```python
from build123d import *

# Parameters (mm, degrees)
F1_DEPTH = 4
F2_R     = 5
F3_R     = 3.99999
F4_DEPTH = 3


# Not quite as in the source:
# - a fillet or chamfer is up to 0.001 mm smaller than in the source, because OpenCascade refuses the exact size
# - a feature names something its author has since deleted; it is built from what else it names


with BuildPart() as f1:
    # F0 (on Front) → F1 (new body)
    with BuildSketch(Plane.XZ):
        with BuildLine():
            Line((-4.5, -6.79), (-4.5, -2.79))
            Line((-4.5, -2.79), (-8, -2.79))
            ThreePointArc((-8, -2.79), (-10.5, -5.29), (-13, -2.79))
            Line((-13, -2.79), (-14.5, -2.79))
            Line((-14.5, -2.79), (-14.5, -6.79))
            Line((-14.5, -6.79), (-4.5, -6.79))
        make_face()
        with BuildLine():
            ThreePointArc((-13, -2.79), (-10.5, -5.29), (-8, -2.79))
            Line((-8, -2.79), (-13, -2.79))
        make_face()
        with BuildLine():
            Line((-3.5307081443, -2.79), (-4.5, -2.79))
            Line((-4.5, -2.79), (-4.5, -6.79))
            Line((-4.5, -6.79), (-3.5307081443, -6.79))
            ThreePointArc((-3.5307081443, -6.79), (-1.9615045246, -5.53), (0, -5.08))
            Line((0, -5.08), (0, -4.5))
            ThreePointArc((0, -4.5), (-1.9615045246, -4.05), (-3.5307081443, -2.79))
        make_face()
        with BuildLine():
            ThreePointArc((4.5, 0), (3.1819805153, 3.1819805153), (0, 4.5))
            ThreePointArc((0, 4.5), (-3.1819805153, 3.1819805153), (-4.5, 0))
            ThreePointArc((-4.5, 0), (-4.2507756145, -1.4767893131), (-3.5307081443, -2.79))
            Line((-3.5307081443, -2.79), (-2.8663391286, -2.79))
            ThreePointArc((-2.8663391286, -2.79), (-1.5057628442, 3.7057628442), (4, 0))
            ThreePointArc((4, 0), (2.8284271247, -2.8284271247), (0, -4))
            Line((0, -4), (0, -4.5))
            ThreePointArc((0, -4.5), (2.2405062847, -3.9025801194), (3.8861134595, -2.2689473726))
            ThreePointArc((3.8861134595, -2.2689473726), (4.3438180537, -1.1752636794), (4.5, 0))
        make_face()
        with BuildLine():
            Line((-2.8663391286, -2.79), (-3.5307081443, -2.79))
            ThreePointArc((-3.5307081443, -2.79), (-1.9615045246, -4.05), (0, -4.5))
            Line((0, -4.5), (0, -4))
            ThreePointArc((0, -4), (-1.5556349186, -3.6851051545), (-2.8663391286, -2.79))
        make_face()
        with BuildLine():
            ThreePointArc((0, -5.08), (-1.9615045246, -5.53), (-3.5307081443, -6.79))
            Line((-3.5307081443, -6.79), (-2.8663391286, -6.79))
            ThreePointArc((-2.8663391286, -6.79), (-1.5556349186, -5.8948948455), (0, -5.58))
            Line((0, -5.58), (0, -5.08))
        make_face()
        with BuildLine():
            ThreePointArc((4.5, -9.58), (4.3438180596, -8.4047363422), (3.886113482, -7.3110526659))
            ThreePointArc((3.886113482, -7.3110526659), (2.240506304, -5.6774198917), (0, -5.08))
            Line((0, -5.08), (0, -5.58))
            ThreePointArc((0, -5.58), (2.8284271247, -6.7515728753), (4, -9.58))
            ThreePointArc((4, -9.58), (-1.5057628442, -13.2857628442), (-2.8663391286, -6.79))
            Line((-2.8663391286, -6.79), (-3.5307081443, -6.79))
            ThreePointArc((-3.5307081443, -6.79), (-4.2507756145, -8.1032106869), (-4.5, -9.58))
            ThreePointArc((-4.5, -9.58), (-3.1819805153, -12.7619805153), (0, -14.08))
            ThreePointArc((0, -14.08), (3.1819805153, -12.7619805153), (4.5, -9.58))
        make_face()
        with BuildLine():
            Line((-3.5307081443, -6.79), (-4.5, -6.79))
            Line((-4.5, -6.79), (-4.5, -9.58))
            ThreePointArc((-4.5, -9.58), (-4.2507756145, -8.1032106869), (-3.5307081443, -6.79))
        make_face()
        with BuildLine():
            ThreePointArc((-3.5307081443, -2.79), (-4.2507756145, -1.4767893131), (-4.5, 0))
            Line((-4.5, 0), (-4.5, -2.79))
            Line((-4.5, -2.79), (-3.5307081443, -2.79))
        make_face()
        with BuildLine():
            ThreePointArc((3.886113482, -7.3110526659), (3.2040173086, -4.7900000223), (3.8861134595, -2.2689473726))
            ThreePointArc((3.8861134595, -2.2689473726), (2.2405062847, -3.9025801194), (0, -4.5))
            Line((0, -4.5), (0, -5.08))
            ThreePointArc((0, -5.08), (2.240506304, -5.6774198917), (3.886113482, -7.3110526659))
        make_face()
    extrude(amount=F1_DEPTH)

    # F2
    f2_edges = [f1.edges().sort_by_distance(p)[0] for p in [
        (-4.5, -2, -2.79),
        (-4.5, -2, -6.79),
    ]]
    fillet(f2_edges, radius=F2_R)

    # F3 (radius 4 in the source; OpenCascade refuses exactly that, so slightly less here)
    f3_edges = [f1.edges().sort_by_distance(p)[0] for p in [
        (-14.5, -2, -6.79),
    ]]
    fillet(f3_edges, radius=F3_R)

    # F0 (on Front) → F4 (cut)
    with BuildSketch(Plane.XZ):
        with BuildLine():
            ThreePointArc((-13, -2.79), (-10.5, -5.29), (-8, -2.79))
            Line((-8, -2.79), (-13, -2.79))
        make_face()
        with BuildLine():
            Line((-13, -2.79), (-8, -2.79))
            ThreePointArc((-8, -2.79), (-10.5, -0.29), (-13, -2.79))
        make_face()
    extrude(amount=F4_DEPTH, mode=Mode.SUBTRACT)


solid = f1.part
```
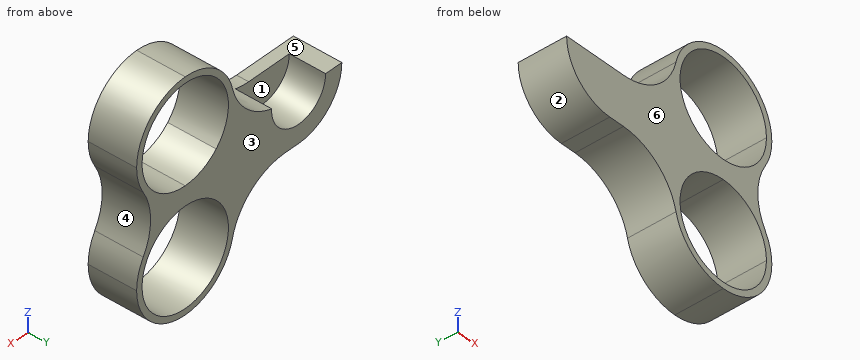
CAD build for the part. Positions are in the model's coordinates, mm. Face numbers are marked on the shaded views. A direction names the side the tool comes from. Round coordinates to 2 decimals unless told otherwise and drop trailing zeros. Order: outer loops, then holes, each group sorted by start corner. A loop starts at its lowest first (then second) coordinate and runs counter-clockwise, first axis right, second up.
Item 1: Saw through at D-D on y = -3.45. State how many separate pieces and enclosed holes the cut face has, then the cut area to 3 significant figures.
Item 2: Saw through at A-A on z = -6. Write the cut outline in (x, y), then the cut area to 3 significant figures.
Item 3: Tool access for the marked faces 5 and 6: list every direction of +Z, -Z, +X, -X, +Y, -Y with a clear straight run to the whole face (end or side of a thin tool).
Item 4: Mould opens along X. For the marked faces 1, 2, 3 and 4 say: pulls with the +X half, pulls with the -X half, needs draft (parallel to the pull), parting line crosses it, or undercut.
Item 5: Saw through at C-C on z = -3.25. Write the cut outline in (x, y).
Item 6: Pin check, flat tips, straight feed: pin 1 (1 mm diameter, centred on x = -9.5, z = -2, fed in from -Y); pin 2 (1.5 mm diameter, centred on x = -5.5, y = -2.5, fed in from -Z). Stop position of each tip, or through.
Item 7: Probe line 1 along Z through (x, y) = (-1.75, -0.25); line 2 along X through (y, z) = (-2.55, -3); line 3 along Z through (x, y) = (-3.5, -3.6). List the from-to ranges inside material, lowest first.
Item 8: Saw through at B-B on x = 1. Write the cut outline in (y, z).
Reported:
1. separate pieces: 1
1. enclosed holes: 2
1. area: 88.3 mm2
2. outline: (-12.89, -4) - (-1.78, -4) - (-1.78, 0) - (-12.89, 0) - close; (1.78, -4) - (3.35, -4) - (3.35, 0) - (1.78, 0) - close
2. area: 50.7 mm2
3. face 5: +Z, -X, +Y, -Y
3. face 6: +Z, -Z, +X, -X, -Y
4. face 1: undercut
4. face 2: pulls with the -X half
4. face 3: needs draft
4. face 4: pulls with the +X half
5. outline: (-14.47, -4) - (-2.33, -4) - (-2.33, 0) - (-8.04, 0) - (-8.04, -3) - (-12.96, -3) - (-12.96, 0) - (-14.47, 0) - close; (2.33, -4) - (3.45, -4) - (3.45, 0) - (2.33, 0) - close
6. pin 1: passes through
6. pin 2: stops at z = -9.59
7. line 1: z = -13.73 to -13.18, -5.98 to -3.6, 3.6 to 4.15
7. line 2: x = -14.49 to -12.99, -8.01 to -2.65, 2.65 to 3.54
7. line 3: z = -12.41 to -11.52, -7.64 to -1.94, 1.94 to 2.83
8. outline: (-4, -13.97) - (0, -13.97) - (0, -13.45) - (-4, -13.45) - close; (-4, -5.71) - (0, -5.71) - (0, -3.87) - (-4, -3.87) - close; (-4, 3.87) - (0, 3.87) - (0, 4.39) - (-4, 4.39) - close
